```python
from build123d import *

# Parameters (mm, degrees)
BOSS_EXTRUDE1_DEPTH              = 5.334
FILLET1_R                        = 0.508
SKETCH2_R                        = 4.572
CUT_EXTRUDE1_DEPTH               = 0.254
CUT_EXTRUDE2_DEPTH               = 0.127
BOSS_EXTRUDE2_DEPTH              = 1.5875
F_56_0_0465_DIAMETER_HOLE1_D     = 1.1811
F_56_0_0465_DIAMETER_HOLE1_DEPTH = 5.08


with BuildPart() as part:
    # Sketch1 → Boss-Extrude1 (new body)
    with BuildSketch(Plane.XY):
        with BuildLine():
            Line((4.362446893, 5.156199954), (-4.362446893, 5.156199954))
            ThreePointArc((-4.362446893, 5.156199954), (-4.923713797, 4.923718126), (-5.156199954, 4.362453015))
            Line((-5.156199954, 4.362453015), (-5.156199954, -4.362453015))
            ThreePointArc((-5.156199954, -4.362453015), (-4.923714856, -4.923717067), (-4.362449887, -5.156199954))
            Line((-4.362449887, -5.156199954), (4.362449887, -5.156199954))
            ThreePointArc((4.362449887, -5.156199954), (4.92371702, -4.923714903), (5.156199954, -4.362446893))
            Line((5.156199954, -4.362446893), (5.156199954, 4.362446893))
            ThreePointArc((5.156199954, 4.362446893), (4.923715961, 4.923715962), (4.362446893, 5.156199954))
        make_face()
    extrude(amount=-BOSS_EXTRUDE1_DEPTH)

    # Fillet1
    fillet1_edges = [part.edges().sort_by_distance(p)[0] for p in [
        (0, 5.156199954, 0),
        (4.923715961, 4.923715962, 0),
        (5.156199954, 0, 0),
        (4.92371702, -4.923714903, 0),
        (0, -5.156199954, 0),
        (-4.923714856, -4.923717067, 0),
        (-5.156199954, 0, 0),
        (-4.923713797, 4.923718126, 0),
    ]]
    fillet(fillet1_edges, radius=FILLET1_R)

    # Sketch2 → Cut-Extrude1 (cut)
    with BuildSketch(Plane.XY):
        Circle(SKETCH2_R)
    extrude(amount=-CUT_EXTRUDE1_DEPTH, mode=Mode.SUBTRACT)

    # Sketch3 → Cut-Extrude2 (cut)
    with BuildSketch(Plane.XY.offset(-0.254)):
        with BuildLine():
            Line((-0.254, 4.564938992), (-0.254, -4.564938992))
            ThreePointArc((-0.254, -4.564938992), (0, -4.572), (0.254, -4.564938992))
            Line((0.254, -4.564938992), (0.254, 4.564938992))
            ThreePointArc((0.254, 4.564938992), (0, 4.572), (-0.254, 4.564938992))
        make_face()
    extrude(amount=-CUT_EXTRUDE2_DEPTH, mode=Mode.SUBTRACT)

    # Sketch4 → Boss-Extrude2 (add)
    with BuildSketch(Plane(origin=(0, 0, -5.334), x_dir=(-1, 0, 0), z_dir=(0, 0, -1))):
        with BuildLine():
            Line((-5.918199954, 4.362443955), (-5.918199954, -4.362446893))
            ThreePointArc((-5.918199954, -4.362446893), (-5.462532364, -5.462530293), (-4.362449822, -5.918199954))
            Line((-4.362449822, -5.918199954), (4.362449887, -5.918199954))
            ThreePointArc((4.362449887, -5.918199954), (5.462529184, -5.462533474), (5.918199954, -4.362455953))
            Line((5.918199954, -4.362455953), (5.918199954, 4.362453015))
            ThreePointArc((5.918199954, 4.362453015), (5.462528126, 5.462534532), (4.362443955, 5.918199954))
            Line((4.362443955, 5.918199954), (-4.362443955, 5.918199954))
            ThreePointArc((-4.362443955, 5.918199954), (-5.462531329, 5.462531329), (-5.918199954, 4.362443955))
        make_face()
    extrude(amount=BOSS_EXTRUDE2_DEPTH)

    # #56 (0.0465) Diameter Hole1
    with Locations(Plane(origin=(0, 0, -6.9215), x_dir=(-1, 0, 0), z_dir=(0, 0, -1))):
        with Locations((0, 0)):
            Hole(F_56_0_0465_DIAMETER_HOLE1_D / 2, depth=F_56_0_0465_DIAMETER_HOLE1_DEPTH)


solid = part.part
```
For this review, take the finished solid that the model builds, in its own axes (mm). A direction names the side the tool comes from. Coordinates: 2 decimals unless noted, no trailing zeros. Order: outer loops, then holes, each group sorted by start corner. A loop starts at its lowest first (then second) coordinate and runs counter-clockwise, first axis right, second up. Notation, with made-up numbers: (-17, 10) - (-1, 10) arc R29 cw to (-1, 37) - close; hole circle Ø8 at (-5.75, -18). An arc over 180 degrees is marked (long way). Answer as a JSON object with one key per item and string values. Group by question number.
1. The part is to be moulded in two halves that separate along X. For faces 1 (the flat face through (5.156, 0, -3)), 2 (the cylindrical face through (-5.475, 5.45, -6.117)), 3 (the cylindrical face through (0.317, 0.498, -4.346)), 4 (the flat face through (5.34, 0.08, -5.334)), say which applies: pulls with the +X half, pulls with the -X half, needs draft (parallel to the pull), parting line crosses it, or undercut.
2. For probe 1 along Y at (x, z) = (0, -4.1); probe 2 along Y at (x, z) = (0, -5.7); probe 3 along Z at (x, y) = (3.5, -5.5), list the stretches that pass through material, from the lowest coordinate up.
3. We need section A-A on z = -6. State the section outline as (x, y) points, then the cut area to 3 significant figures.
4. Clearance check with flat-ended pins moving along their axes: P1, Ø2, axis at x = 4.5, z = -2, coming from the -Y side; P2, Ø5.5, axis at x = 0, y = 0, coming from the +Z side; P3, Ø2.5, axis at y = 2, z = -4, coming from the +X side; P4, Ø4, axis at y = -2.5, z = -3.5, coming from the -X side. State where each tip first meets the part, or that it passes through.
5. We need section D-D on z = -1. State the section outline as (x, y) points.
6. We need section B-B on y = 0. State the section outline as (x, z) points, then the cut area to 3 significant figures.
7. We need section C-C on x = 0. State the section outline as (y, z) points, then the cut area to 3 significant figures.
8. For faces 5 (the flat face through (0, 5.156, -3)), 6 (the flat face through (0, -5.156, -3)), 7 (the flat face through (0, 0, -1.842)), list the 3-axis set-ups (+Z, -Z, +X, -X, +Y, -Y) from which the entire face can be reached by the end or side of a thin tool; tool diameter is ignored.
Final values:
{
 "1": {"face 1": "pulls with the +X half", "face 2": "pulls with the -X half", "face 3": "undercut", "face 4": "needs draft"},
 "2": {"probe 1": "-5.16 to -0.59, 0.59 to 5.16", "probe 2": "-5.92 to -0.59, 0.59 to 5.92", "probe 3": "-6.92 to -5.33"},
 "3": {"outline": "(-5.92, -4.36) arc R1.56 ccw to (-4.36, -5.92) - (4.36, -5.92) arc R1.56 ccw to (5.92, -4.36) - (5.92, 4.36) arc R1.56 ccw to (4.36, 5.92) - (-4.36, 5.92) arc R1.56 ccw to (-5.92, 4.36) - close; hole circle Ø1.18 at (0, 0)", "area": "137 mm²"},
 "4": {"P1": "y = -5.16", "P2": "z = -0.25", "P3": "x = 5.16", "P4": "x = -5.92"},
 "5": {"outline": "(-5.16, -4.36) arc R0.79 ccw to (-4.36, -5.16) - (4.36, -5.16) arc R0.79 ccw to (5.16, -4.36) - (5.16, 4.36) arc R0.79 ccw to (4.36, 5.16) - (-4.36, 5.16) arc R0.79 ccw to (-5.16, 4.36) - close"},
 "6": {"outline": "(-5.92, -6.92) - (-0.59, -6.92) - (-0.59, -1.84) - (0.59, -1.84) - (0.59, -6.92) - (5.92, -6.92) - (5.92, -5.33) - (5.16, -5.33) - (5.16, -0.51) arc R0.51 ccw to (4.65, 0) - (4.57, 0) - (4.57, -0.25) - (0.25, -0.25) - (0.25, -0.38) - (-0.25, -0.38) - (-0.25, -0.25) - (-4.57, -0.25) - (-4.57, 0) - (-4.65, 0) arc R0.51 ccw to (-5.16, -0.51) - (-5.16, -5.33) - (-5.92, -5.33) - close", "area": "65.3 mm²"},
 "7": {"outline": "(-5.92, -6.92) - (-0.59, -6.92) - (-0.59, -1.84) - (0.59, -1.84) - (0.59, -6.92) - (5.92, -6.92) - (5.92, -5.33) - (5.16, -5.33) - (5.16, -0.51) arc R0.51 ccw to (4.65, 0) - (4.57, 0) - (4.57, -0.38) - (-4.57, -0.38) - (-4.57, 0) - (-4.65, 0) arc R0.51 ccw to (-5.16, -0.51) - (-5.16, -5.33) - (-5.92, -5.33) - close", "area": "64.2 mm²"},
 "8": {"face 5": "+Z, +X, -X, +Y", "face 6": "+Z, +X, -X, -Y", "face 7": "-Z"}
}
